Build history of the part. All positions in model axes, mm. A direction names the side the tool comes from. Give positions to 0.01 mm unless a question says otherwise; leave off trailing zeros. Order: outer loops, then holes, each group sorted by start corner. A loop starts at its lowest first (then second) coordinate and runs counter-clockwise, first axis right, second up. Notation, with made-up numbers: (-24, -12) -> (31, -12) arc R11 ccw to (31, 5) -> close; hole circle Ø8 at (10, 45). An arc over 180 degrees is marked (long way). One line per question, with ' | ' between items. Start each with the question number.
(1) Pull direction X, two halves, no side cores. Call faces 1 (the face through (-1.174, 90, 1)), 2 (the face through (1.076, 90, 5)), 3 (the face through (-13, 91, 3)): +X half, -X half, draft (parallel to the pull), parting line (faces both ways), or undercut.
(2) Which spindle directions (+Z, -Z, +X, -X, +Y, -Y) get a long thin tool onto all of the face, cutting with end or side? Do faces 4 (the face through (-9.174, 90, 1)), 5 (the face through (-5, 47.714, 3)), 6 (the face through (2, 91, 3)), 7 (the face through (-11.424, 91, 5)), 8 (the face through (1, 57, 1.236)). Say none if no direction does.
(3) Pin check, flat tips, straight feed: pin 1 Ø1.3 at (x, y) = (2.5, 90) entering from +Z; pin 2 Ø4 at (x, y) = (-12, 56.5) entering from -Z; pin 3 Ø3 at (x, y) = (2, 56.5) entering from -Z. Stop position of each tip, or through.
(4) Cut at B-B (z = 6). Give the cut face in (x, y).
(5) Drill centre lines: L1, parallel to Z at x = -2.5, y = 103; L2, parallel to X at y = 99, z = 3.5; L3, parallel to Z at x = -11.75, y = 111.5. Where is each one in solid material? Low to high. Write a range as from..to.
(6) Cut at C-C (x = -5.5). Give the cut face in (y, z).
(7) Cut at A-A (y = 92.5). Give the cut face in (x, z).
from build123d import *

# Parameters (mm, degrees)
F0_W     = 17.7
F0_H     = 86
F1_DEPTH = 3
F3_DEPTH = 4
F5_DEPTH = 86
F7_DEPTH = 25


with BuildPart() as f1:
    # F0 (on Top) → F1 (new body)
    with BuildSketch(Plane.XY):
        with Locations((-5.174149, 90.714084)):
            Rectangle(F0_W, F0_H)
    extrude(amount=F1_DEPTH)

    # F2 (on face) → F3 (join)
    with BuildSketch(Plane.XY.offset(3)):
        Polygon((-11.424149, 47.714084), (-5.174149, 47.714084), (1.075851, 47.714084), (1.075851, 133.714084), (-11.424149, 133.714084), align=None)
    extrude(amount=F3_DEPTH)

    # F4 (on face) → F5 (cut)
    with BuildSketch(Plane.XZ.offset(-47.714084)):
        Polygon((-9.174149, 0), (-5.174149, 0), (-1.174149, 0), (-1.174149, 1.5), (-9.174149, 1.5), align=None)
    extrude(amount=-F5_DEPTH, mode=Mode.SUBTRACT)

    # F6 (on face) → F7 (cut)
    with BuildSketch(Plane(origin=(-14.024149, 0, 0), x_dir=(0, -1, 0), z_dir=(-1, 0, 0))):
        Polygon((-60.08194, 0), (-53.346284, 0), (-54.954443, 1.236051), (-58.471706, 1.236051), align=None)
    extrude(amount=-F7_DEPTH, mode=Mode.SUBTRACT)


solid = f1.part
Result set:
1) face 1: undercut | face 2: +X half | face 3: draft
2) face 4: -Z, +Y, -Y | face 5: +Z, -Z, +X, -X, -Y | face 6: +Z, +X, +Y, -Y | face 7: +Z, -X, +Y, -Y | face 8: -Z, +X, -X
3) pin 1: stops at z = 3 | pin 2: stops at z = 0.89 | pin 3: stops at z = 1.24
4) outline: (-11.42, 47.71) -> (1.08, 47.71) -> (1.08, 133.71) -> (-11.42, 133.71) -> close
5) L1: z = 1.5..7 | L2: x = -11.42..1.08 | L3: z = 0..3
6) outline: (47.71, 1.5) -> (133.71, 1.5) -> (133.71, 7) -> (47.71, 7) -> close
7) outline: (-14.02, 0) -> (-9.17, 0) -> (-9.17, 1.5) -> (-1.17, 1.5) -> (-1.17, 0) -> (3.68, 0) -> (3.68, 3) -> (1.08, 3) -> (1.08, 7) -> (-11.42, 7) -> (-11.42, 3) -> (-14.02, 3) -> close
